The listing builds one solid part. Answer for the finished solid, in the listing's coordinates (mm). Face numbers are marked on the shaded views. A direction names the side the tool comes from. Round coordinates to 2 decimals unless told otherwise and drop trailing zeros. Write each loop counter-clockwise with the first axis right and the second up, starting at its lowest first coordinate (ties: lowest second). Pieces come first, ordered by that corner, then holes. Notation, with made-up numbers: (76, -3) - (87, -3) arc R29 cw to (87, 33) - close; hole circle Ø5 at (75.5, 80). An arc over 180 degrees is marked (long way). Answer in a Markdown table with one row per item.
from build123d import *

# Parameters (mm, degrees)
CROQUIS1_R              = 100
SALIENTE_EXTRUIR1_DEPTH = 50
CROQUIS2_W              = 300
CROQUIS2_H              = 100
SALIENTE_EXTRUIR2_DEPTH = 150
CORTAR_EXTRUIR1_DEPTH   = 150
CROQUIS6_R              = 100
SALIENTE_EXTRUIR3_DEPTH = 20


with BuildPart() as part:
    # Croquis1 → Saliente-Extruir1 (new body)
    with BuildSketch(Plane.XY):
        Circle(CROQUIS1_R)
    extrude(amount=SALIENTE_EXTRUIR1_DEPTH)

    # Croquis2 → Saliente-Extruir2 (add)
    with BuildSketch(Plane.XY.offset(50)):
        Rectangle(CROQUIS2_W, CROQUIS2_H)
    extrude(amount=SALIENTE_EXTRUIR2_DEPTH)

    # Croquis3 → Cortar-Extruir1 (cut)
    with BuildSketch(Plane.XZ.offset(50)):
        Polygon((-100, 162.170416567), (-50, 162.170416567), (-50, 200), (50, 200), (50, 162.170416567), (100, 162.170416567), (100, 80), (-100, 80), align=None)
    extrude(amount=-CORTAR_EXTRUIR1_DEPTH, mode=Mode.SUBTRACT)

    # Croquis6 → Saliente-Extruir3 (add)
    with BuildSketch(Plane(origin=(0, 0, 0), x_dir=(-1, 0, 0), z_dir=(0, 0, -1))):
        Circle(CROQUIS6_R)
    extrude(amount=SALIENTE_EXTRUIR3_DEPTH)


solid = part.part
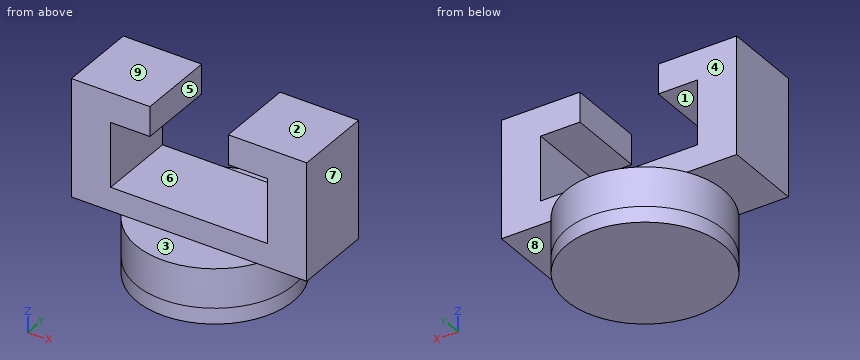
(1) For a pull along Z with two mould halves and no side action, classify the marked faces 6, 7, 8 and 9 as pulls with the +Z half, pulls with the -Z half, needs draft (parallel to the pull), parting line crosses it, or undercut.
Checked values:
| item | result |
|---|---|
| face 6 | undercut |
| face 7 | needs draft |
| face 8 | pulls with the -Z half |
| face 9 | pulls with the +Z half |
(2) Section A-A (z = 173.5) is taken. Give the vertices of the cut face in (x, y), and give its area (3 significant figures).
Checked values:
| item | result |
|---|---|
| outline | (-150, -50) - (-50, -50) - (-50, 50) - (-150, 50) - close; (50, -50) - (150, -50) - (150, 50) - (50, 50) - close |
| area | 20,000 mm2 |
(3) Find the intervals of material crossed by line 1 (X direction, y = 22.5, z = 190.5); line 2 (Z direction, x = 51, y = -30); line 3 (X direction, y = -47.5, z = 120), in increasing order.
Checked values:
| item | result |
|---|---|
| line 1 | x = -150 to -50, 50 to 150 |
| line 2 | z = -20 to 80, 162.17 to 200 |
| line 3 | x = -150 to -100, 100 to 150 |
(4) For the marked faces 1, 2, 3, 4 and 5, determine the directions among +Z, -Z, +X, -X, +Y, -Y from which every point of the face is accessible in a straight line to the end or side of a thin tool.
Checked values:
| item | result |
|---|---|
| face 1 | +Y, -Y |
| face 2 | +Z, +X, -X, +Y, -Y |
| face 3 | +Z, +X, -X, -Y |
| face 4 | +Z, +X, -X, +Y |
| face 5 | +Z, +Y, -Y |
(5) Flat-ended cylindrical pins translate along their axes: pin 1 (3 mm diameter, centred on y = 65, z = 43.5, fed in from -X); pin 2 (3 mm diameter, centred on y = -20, z = 24.5, fed in from -X); pin 3 (19 mm diameter, centred on x = 115.5, y = 20.5, fed in from -Z); pin 4 (8 mm diameter, centred on y = -17.5, z = 49.5, fed in from +X). Find the tip coordinate at first contact, or state that the pin passes through.
Checked values:
| item | result |
|---|---|
| pin 1 | stops at x = -77.25 |
| pin 2 | stops at x = -98.27 |
| pin 3 | stops at z = 50 |
| pin 4 | stops at x = 150 |
(6) Section B-B (x = 70) is taken. Give the vertices of the cut face in (y, z), and give its area (3 significant figures).
Checked values:
| item | result |
|---|---|
| outline | (-71.41, -20) - (71.41, -20) - (71.41, 50) - (50, 50) - (50, 80) - (-50, 80) - (-50, 50) - (-71.41, 50) - close; (-50, 162.17) - (50, 162.17) - (50, 200) - (-50, 200) - close |
| area | 16,800 mm2 |
(7) Section C-C (y = 0) is taken. Give the vertices of the cut face in (x, z).
Checked values:
| item | result |
|---|---|
| outline | (-150, 50) - (-100, 50) - (-100, -20) - (100, -20) - (100, 50) - (150, 50) - (150, 200) - (50, 200) - (50, 162.17) - (100, 162.17) - (100, 80) - (-100, 80) - (-100, 162.17) - (-50, 162.17) - (-50, 200) - (-150, 200) - close |
(8) Section D-D (x = 0) is taken. Give the vertices of the cut face in (y, z).
Checked values:
| item | result |
|---|---|
| outline | (-100, -20) - (100, -20) - (100, 50) - (50, 50) - (50, 80) - (-50, 80) - (-50, 50) - (-100, 50) - close |
